CAD build for the part. Positions are in the model's coordinates, mm. A direction names the side the tool comes from. Give positions to 0.01 mm unless a question says otherwise; leave off trailing zeros. Loops run counter-clockwise (first coordinate to the right, second up) from the corner with the lowest first, then second, coordinate; pieces in that order, holes last.
```python
from build123d import *

# Parameters (mm, degrees)
SKETCH1_W           = 330.2
SKETCH1_H           = 279.4
BOSS_EXTRUDE1_DEPTH = 6.35
SKETCH2_W           = 12.7
SKETCH2_H           = 152.4
CUT_EXTRUDE1_DEPTH  = 217.645770787
SKETCH4_W           = 31.75
SKETCH4_H           = 279.4
CUT_EXTRUDE3_DEPTH  = 217.645770787
CAVITY1_START       = -28.48121296
CAVITY1_OUTLINE_R   = 12.7
CAVITY1_DEPTH       = 23.121998378


# Read off the part's stored shape, not the designer's step: Cavity1
with BuildPart() as part:
    # Sketch1 → Boss-Extrude1 (new, symmetric)
    with BuildSketch(Plane(origin=(0, 0, 0), x_dir=(1, 0, 0), z_dir=(0, 1, 0))):
        Rectangle(SKETCH1_W, SKETCH1_H)
    extrude(amount=BOSS_EXTRUDE1_DEPTH, both=True)

    # Sketch2 → Cut-Extrude1 (cut, through all)
    with BuildSketch(Plane(origin=(0, 6.35, 0), x_dir=(1, 0, 0), z_dir=(0, 1, 0))):
        with Locations((-107.95, 63.5)):
            Rectangle(SKETCH2_W, SKETCH2_H)
        with Locations((107.95, 63.5)):
            Rectangle(SKETCH2_W, SKETCH2_H)
    extrude(amount=-CUT_EXTRUDE1_DEPTH, mode=Mode.SUBTRACT)

    # Sketch4 → Cut-Extrude3 (cut, through all)
    with BuildSketch(Plane(origin=(0, 6.35, 0), x_dir=(1, 0, 0), z_dir=(0, 1, 0))):
        with Locations((-149.225, 0)):
            Rectangle(SKETCH4_W, SKETCH4_H)
        with Locations((149.225, 0)):
            Rectangle(SKETCH4_W, SKETCH4_H)
    extrude(amount=-CUT_EXTRUDE3_DEPTH, mode=Mode.SUBTRACT)

    # Cavity1 outline → Cavity1 (cut)
    with BuildSketch(Plane(origin=(0, 0, 0), x_dir=(0.999972352848875, -0.006960139267425278, -0.0026172503248496305), z_dir=(0.007435962471992497, 0.9359846644758757, 0.3519622342355749)).offset(CAVITY1_START)):
        with Locations((0.653273782, 45.008151356)):
            Circle(CAVITY1_OUTLINE_R)
    extrude(amount=CAVITY1_DEPTH, mode=Mode.SUBTRACT)


solid = part.part
```
1. Drop a flat-ended pin along its axis: pin 1 (4 mm diameter, centred on x = -106, y = 2, fed in from -Z). Give the stop position or say it passes through.
Responses:
pin 1: stops at z = 12.7
2. Saw through at A-A, the plane z = -114.5. List the corners of the cut face in (x, y).
Responses:
outline: (-133.35, -6.35) - (-114.3, -6.35) - (-114.3, 6.35) - (-133.35, 6.35) - close; (-101.6, -6.35) - (101.6, -6.35) - (101.6, 6.35) - (-101.6, 6.35) - close; (114.3, -6.35) - (133.35, -6.35) - (133.35, 6.35) - (114.3, 6.35) - close
3. Tool access for faces 4 (the face through (-2, 6.35, -2)), 5 (the face through (-114.3, 0, -62)): list every direction of +Z, -Z, +X, -X, +Y, -Y with a clear straight run to the whole face (end or side of a thin tool).
Responses:
face 4: +Z, -Z, +X, -X, +Y
face 5: -Z, +Y, -Y
4. Saw through at B-B, the plane z = -40.5. Count the separate pieces of the cut face and the enclosed holes in it, and give its area (3 significant figures).
Responses:
separate pieces: 4
enclosed holes: 0
area: 2,800 mm2
5. Probe line 1 along X through (y, z) = (-1.5, -63); line 2 along X through (y, z) = (3.75, -37); line 3 along X through (y, z) = (5.25, -54.5). List the from-to ranges inside material, lowest first.
Responses:
line 1: x = -133.35 to -114.3, -101.6 to 101.6, 114.3 to 133.35
line 2: x = -133.35 to -114.3, -101.6 to -8.32, 9.49 to 101.6, 114.3 to 133.35
line 3: x = -133.35 to -114.3, -101.6 to -9.43, 10.53 to 101.6, 114.3 to 133.35
6. Pull direction X, two halves, no side cores. Call faces 1 (the face through (-2, 0, 139.7)), 2 (the face through (-133.35, 0, 2)), 3 (the face through (114.3, 0, -62)): released by +X, released by -X, zero draft, split by the parting line, or undercut.
Responses:
face 1: zero draft
face 2: released by -X
face 3: undercut
